Input: part model. Units: mm. Frame: model coordinates. A direction names the side the tool comes from. Coordinates: 2 decimals unless noted, no trailing zeros. Loops run counter-clockwise (first coordinate to the right, second up) from the corner with the lowest first, then second, coordinate; pieces in that order, holes last.
(1) Section B-B, the plane z = 7.75. Return loops of the section in (x, y).
(2) Section C-C, the plane x = 34. Return loops of the section in (y, z), then the cut area to 3 significant figures.
(3) Line query: L1, parallel to Y at x = 0, z = 7.25; L2, parallel to X at y = -7.75, z = 2; L3, parallel to X at y = -8, z = 1.25. Output: solid intervals per line, ascending.
(4) Contact query for flat-ended pins moving along their axis: P1, Ø1, axis at y = -3, z = 0, coming from the -X side; P2, Ø6.5, axis at x = -3, y = 3.5, coming from the +Z side; P3, Ø2, axis at x = 2.5, z = -2, coming from the -Y side; P4, Ø1, axis at x = -0.5, z = -1.5, coming from the +Y side. Output: stop coordinate, or through.
(5) Section D-D, the plane x = 59. Return loops of the section in (y, z), then the cut area to 3 significant figures.
(6) Section A-A, the plane z = 3.5. Return loops of the section in (x, y).
(7) Mould query, pull axis X, two halves, no side actions, for faces 1 (the face through (89.95, -15.44, 0.07)), 2 (the face through (12.992, -3.712, 0.07)), 3 (the face through (92.31, -10.2, 0.07)). Classes: released by +X, released by -X, zero draft, split by the parting line, or undercut.
(8) Set-up query: faces 4 (the face through (0, 0, 5)), 5 (the face through (1, -11, 8.75)), 6 (the face through (75.213, -9.847, 0.07)), 7 (the face through (33, 7, 0)). Return all of +Z, -Z, +X, -X, +Y, -Y with unobstructed straight access to the full face (end or side cutting, diameter ignored); none if empty.
```python
from build123d import *

# Parameters (mm, degrees)
BOSS_EXTRU_1_DEPTH  = 5
CONG_4_R            = 5
CONG_3_R            = 15
CONG_6_R            = 5
SKETCH4_R           = 0.75
CUT_EXTRUDE5_DEPTH  = 95.659933807
BOSS_EXTRUDE1_START = -13.75
SKETCH5_R           = 12.5
SKETCH5_R_2         = 10.5
BOSS_EXTRUDE1_DEPTH = 3.75


with BuildPart() as part:
    # Esquisse1 → Boss.-Extru.1 (new, symmetric)
    with BuildSketch(Plane.XY):
        with BuildLine():
            Line((10.356157589, 7), (58.01560049, 7))
            Line((58.01560049, 7), (94.472218138, -10))
            Line((94.472218138, -10), (91.091272045, -17.250462296))
            Line((91.091272045, -17.250462296), (60.53105703, -3))
            Line((60.53105703, -3), (12.1346611, -3))
            ThreePointArc((12.1346611, -3), (-12.306877399, -2.188782466), (10.356157589, 7))
        make_face()
    extrude(amount=BOSS_EXTRU_1_DEPTH, both=True)

    # Congé4
    cong_4_edges = [part.edges().sort_by_distance(p)[0] for p in [
        (12.1346611, -3, 0),
        (10.356157589, 7, 0),
    ]]
    fillet(cong_4_edges, radius=CONG_4_R)

    # Congé3
    cong_3_edges = [part.edges().sort_by_distance(p)[0] for p in [
        (60.53105703, -3, 0),
        (58.01560049, 7, 0),
    ]]
    fillet(cong_3_edges, radius=CONG_3_R)

    # Congé6
    # the kernel refuses this fillet: 5 mm, written as the material it takes off along each edge
    with BuildSketch(Plane(origin=(94.472218138, -10, 17.5), x_dir=(-0.906307787036649, 0.4226182617407012, 0), z_dir=(0, 0, -1)), Plane(origin=(91.091272045, -17.250462296, 17.5), x_dir=(0.4226182617407007, 0.9063077870366493, 0), z_dir=(0, 0, -1))) as cong_6_piece_1:
        with BuildLine():
            CenterArc((CONG_6_R, -CONG_6_R), CONG_6_R, 90, 90)
            Line((0, -CONG_6_R), (0, 0))
            Line((0, 0), (CONG_6_R, 0))
        make_face()
    extrude(amount=35, mode=Mode.SUBTRACT)

    # Sketch4 → Cut-Extrude5 (cut, through all)
    with BuildSketch(Plane(origin=(0, 0, -5), x_dir=(-1, 0, 0), z_dir=(0, 0, -1))):
        with Locations((-1.410466322, 7.874679978)):
            Circle(SKETCH4_R)
        with Locations((7.874679978, 1.410466322)):
            Circle(SKETCH4_R)
        with Locations((1.410466322, -7.874679978)):
            Circle(SKETCH4_R)
        with Locations((-7.874679978, -1.410466322)):
            Circle(SKETCH4_R)
    extrude(amount=-CUT_EXTRUDE5_DEPTH, mode=Mode.SUBTRACT)

    # Sketch5 → Boss-Extrude1 (add)
    with BuildSketch(Plane(origin=(0, 0, -5), x_dir=(-1, 0, 0), z_dir=(0, 0, -1)).offset(BOSS_EXTRUDE1_START)):
        with Locations(Location((0, 0, 0), (0, 0, 136.708192407))):
            Circle(SKETCH5_R)
        with Locations(Location((0, 0, 0), (0, 0, 180))):
            Circle(SKETCH5_R_2, mode=Mode.SUBTRACT)
    extrude(amount=BOSS_EXTRUDE1_DEPTH)


solid = part.part
```
Report:
1. outline: circle Ø25 at (0, 0); hole circle Ø21 at (0, 0)
2. outline: (-3, -5) - (7, -5) - (7, 5) - (-3, 5) - close
2. area: 100 mm2
3. L1: y = -12.5 to -10.5, 10.5 to 12.5
3. L2: x = -9.81 to -2.15, -0.67 to 9.81, 70.72 to 89.65
3. L3: x = -9.6 to -2.15, -0.67 to 9.6, 71.25 to 90.17
4. P1: stops at x = -12.25
4. P2: stops at z = 5
4. P3: stops at y = -12.41
4. P4: stops at y = 12.5
5. outline: (-3.11, -5) - (6.37, -5) - (6.37, 5) - (-3.11, 5) - close
5. area: 94.8 mm2
6. outline: (9.1, 8.57) arc R12.5 ccw (long way) to (11.12, -5.71) arc R5 cw to (15.56, -3) - (57.21, -3) arc R15 cw to (63.54, -4.41) - (86.56, -15.14) arc R5 ccw to (92.69, -13.58) arc R5 ccw to (89.94, -7.89) - (61.03, 5.59) arc R15 ccw to (54.69, 7) - (12.74, 7) arc R5 cw to start; hole circle Ø1.5 at (-7.87, 1.41); hole circle Ø1.5 at (-1.41, -7.87); hole circle Ø1.5 at (1.41, 7.87); hole circle Ø1.5 at (7.87, -1.41)
7. face 1: split by the parting line
7. face 2: undercut
7. face 3: released by +X
8. face 4: +Z
8. face 5: +Z, +X, -X, +Y, -Y
8. face 6: +Z, -Z, -Y
8. face 7: +Z, -Z, +X, +Y
